```python
from build123d import *

# Parameters (mm, degrees)
BOSS_EXTRUDE1_DEPTH = 42
SKETCH2_R           = 12
SKETCH2_R_2         = 1.5
CUT_EXTRUDE1_DEPTH  = 5
SKETCH3_R           = 2
CUT_EXTRUDE2_DEPTH  = 5
CHAMFER1_SIZE       = 2
CHAMFER2_SIZE       = 1
FILLET1_R           = 4


with BuildPart() as part:
    # Sketch1 → Boss-Extrude1 (new body)
    with BuildSketch(Plane(origin=(0, 0, 0), x_dir=(1, 0, 0), z_dir=(0, 1, 0))):
        Polygon((0, 0), (0, 42), (-20, 42), (-20, 46), (4, 46), (4, 0), align=None)
    extrude(amount=BOSS_EXTRUDE1_DEPTH)

    # Sketch2 → Cut-Extrude1 (cut, through all)
    with BuildSketch(Plane.ZY):
        with Locations((-21, 21)):
            Circle(SKETCH2_R)
        with Locations((-36.5, 36.5)):
            Circle(SKETCH2_R_2)
        with Locations((-5.5, 36.5)):
            Circle(SKETCH2_R_2)
        with Locations((-5.5, 5.5)):
            Circle(SKETCH2_R_2)
        with Locations((-36.5, 5.5)):
            Circle(SKETCH2_R_2)
    extrude(amount=-CUT_EXTRUDE1_DEPTH, mode=Mode.SUBTRACT)

    # Sketch3 → Cut-Extrude2 (cut, through all)
    with BuildSketch(Plane.XY.offset(-42)):
        with Locations((-10, 32)):
            Circle(SKETCH3_R)
        with Locations((-10, 10)):
            Circle(SKETCH3_R)
    extrude(amount=-CUT_EXTRUDE2_DEPTH, mode=Mode.SUBTRACT)

    # Chamfer1
    chamfer1_edges = [part.edges().sort_by_distance(p)[0] for p in [
        (-12, 32, -42),
        (-12, 10, -42),
    ]]
    chamfer(chamfer1_edges, length=CHAMFER1_SIZE)

    # Chamfer2
    chamfer2_edges = [part.edges().sort_by_distance(p)[0] for p in [
        (0, 21, -33),
    ]]
    chamfer(chamfer2_edges, length=CHAMFER2_SIZE)

    # Fillet1
    fillet1_edges = [part.edges().sort_by_distance(p)[0] for p in [
        (4, 21, -46),
        (-20, 42, -44),
        (2, 42, 0),
        (-20, 0, -44),
        (2, 0, 0),
    ]]
    fillet(fillet1_edges, radius=FILLET1_R)


solid = part.part
```
Geometry check sheet. Reference: the model listing, model coordinates, mm. A direction names the side the tool comes from. Round coordinates to 2 decimals unless told otherwise and drop trailing zeros. Write each loop counter-clockwise with the first axis right and the second up, starting at its lowest first coordinate (ties: lowest second). Pieces come first, ordered by that corner, then holes. Notation, with made-up numbers: (81, -5) - (139, -5) arc R30 cw to (139, 20) - close; hole circle Ø5 at (74, 81). An arc over 180 degrees is marked (long way). Write each question's results on one line, items separated by ' | '.
(1) Sectioned sample at B-B, the plane y = 21. Enter the section's corners in (x, z).
Computed:
outline: (-20, -46) - (0, -46) arc R4 ccw to (4, -42) - (4, -33) - (1, -33) - (0, -34) - (0, -42) - (-20, -42) - close; (0, -8) - (1, -9) - (4, -9) - (4, 0) - (0, 0) - close
(2) Draft check along X on faces 3 (the face through (-18.797, 40.859, -44.028)), 4 (the face through (-10, 30, -45)), 5 (the face through (-10, 12, -45)), 6 (the face through (2.859, 21.294, -44.797)). Enter one of: pulls with the +X half, pulls with the -X half, needs draft (parallel to the pull), parting line crosses it, or undercut.
Computed:
face 3: pulls with the -X half | face 4: undercut | face 5: undercut | face 6: pulls with the +X half
(3) Sectioned sample at A-A, the plane z = -5.5. Enter the section's corners in (x, y).
Computed:
outline: (0, 0) - (4, 0) - (4, 4) - (0, 4) - close; (0, 7) - (4, 7) - (4, 35) - (0, 35) - close; (0, 38) - (4, 38) - (4, 42) - (0, 42) - close
(4) Sectioned sample at C-C, the plane x = -15. Enter the section's corners in (y, z).
Computed:
outline: (0, -46) - (42, -46) - (42, -42) - (0, -42) - close
(5) Set-up check for faces 1 (the face through (-10, 21, -42)), 2 (the face through (1.972, 40.797, -1.141)): record each of +Z, -Z, +X, -X, +Y, -Y from which the full face is reachable in a straight line by a thin tool's end or side.
Computed:
face 1: +Z, -X, +Y, -Y | face 2: +Z, +X, -X, +Y
(6) Depth check by flat-ended pin: pin 1 Ø2.5 at (y, z) = (5.5, -36.5) entering from -X; pin 2 Ø2 at (y, z) = (15.5, -37.5) entering from -X; pin 3 Ø1 at (x, y) = (1.5, 6) entering from -Z; pin 4 Ø8 at (x, y) = (-11.5, 31.5) entering from +Z. Enter the tip coordinate at first touch or a pass-through.
Computed:
pin 1: passes through | pin 2: stops at x = 0 | pin 3: stops at z = -45.87 | pin 4: stops at z = -42
(7) Sectioned sample at D-D, the plane y = 10. Count the separate pieces of the cut face and the enclosed holes in it, plus the area to 3 significant figures.
Computed:
separate pieces: 3 | enclosed holes: 0 | area: 200 mm^2
(8) Thickness scan on probe 1 along Y at (x, z) = (2.55, -5.5); probe 2 along Y at (x, z) = (-9, -42.5); probe 3 along X at (y, z) = (30.5, -30). Record the ranges inside material, lowest first. Write a range as from..to.
Computed:
probe 1: y = 0..4, 7..35, 38..42 | probe 2: y = 0..6.65, 13.35..28.65, 35.35..42 | probe 3: x = 0..4
